Could you check a few things on this model? Use its own coordinates, in mm. Face numbers are marked on the shaded views. Give positions to 0.01 mm unless a question says otherwise; leave off trailing zeros. Loops run counter-clockwise (first coordinate to the right, second up) from the corner with the lowest first, then second, coordinate; pieces in that order, holes last.
1. Imagine slicing it at A-A (z = 8). List the corners of the cut face in (x, y) for me, plus the area to 3 significant figures.
2. I need wall thicknesses on line 1 along Y through (x, z) = (0, 12.2); line 2 along Y through (x, z) = (0, 7.75); line 3 along Z through (x, y) = (4.25, -5.5). Which ranges of each line are inside material? Lowest first, please.
3. Thinking about a two-plate mould opening in X: for the marked faces 1, 2 and 3, which applies, +X half, -X half, draft (parallel to the pull), parting line (faces both ways), or undercut?
4. For P1, Ø12, axis at x = -2, y = -3, coming from the +Z side; P2, Ø4, axis at y = 6.5, z = 2, coming from the +X side; P3, Ø4, axis at x = 4.5, z = 10.5, coming from the -Y side; P4, Ø11, axis at x = 0, y = 0, coming from the +Z side, each with a flat end and sliding along its axis, tell me the tip position at first contact or that it passes through.
```python
from build123d import *

# Parameters (mm, degrees)
F0_R     = 11
F0_R_2   = 8
F0_R_3   = 4.25
F1_DEPTH = 11
F2_DEPTH = 14
F3_SIZE  = 1
F4_R     = 0.5
F5_SIZE  = 1


with BuildPart() as f1:
    # F0 (on Top) → F1 (new body)
    with BuildSketch(Plane.XY):
        Circle(F0_R)
        Circle(F0_R_2, mode=Mode.SUBTRACT)
        Circle(F0_R_2)
        Circle(F0_R_3, mode=Mode.SUBTRACT)
    extrude(amount=F1_DEPTH)

    # F0 (on Top) → F2 (join)
    with BuildSketch(Plane.XY):
        Circle(F0_R)
        Circle(F0_R_2, mode=Mode.SUBTRACT)
    extrude(amount=F2_DEPTH)

    # F3
    f3_edges = [f1.edges().sort_by_distance(p)[0] for p in [
        (-8, 0, 14),
    ]]
    chamfer(f3_edges, length=F3_SIZE)

    # F4
    f4_edges = [f1.edges().sort_by_distance(p)[0] for p in [
        (-9, 0, 14),
        (-8, 0, 13),
        (-11, 0, 14),
        (-8, 0, 11),
        (-4.25, 0, 11),
    ]]
    fillet(f4_edges, radius=F4_R)

    # F5
    f5_edges = [f1.edges().sort_by_distance(p)[0] for p in [
        (-11, 0, 0),
        (-4.25, 0, 0),
    ]]
    chamfer(f5_edges, length=F5_SIZE)


solid = f1.part
```
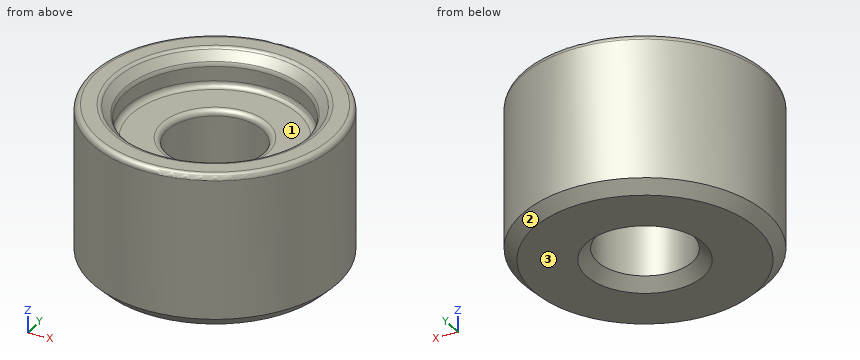
Derived:
1. outline: circle Ø22 at (0, 0); hole circle Ø8.5 at (0, 0)
1. area: 323 mm2
2. line 1: y = -11 to -8, 8 to 11
2. line 2: y = -11 to -4.25, 4.25 to 11
2. line 3: z = 0 to 11
3. face 1: undercut
3. face 2: parting line
3. face 3: draft
4. P1: stops at z = 14
4. P2: stops at x = 10.04
4. P3: stops at y = -10.71
4. P4: stops at z = 11
